```python
from build123d import *

# Parameters (mm, degrees)
EXTRUDE_1_DEPTH     = 5
FILLET_1_R          = 3
SKETCH_11_R         = 2
CUT_EXTRUDE_6_DEPTH = 88.5
SKETCH_12_R         = 2
CUT_EXTRUDE_7_DEPTH = 88.5
SKETCH_13_R         = 1.5
SKETCH_13_R_2       = 9
SKETCH_13_W         = 9.590692188
SKETCH_13_H         = 23
CUT_EXTRUDE_8_DEPTH = 10


with BuildPart() as part:
    # 스케치1 → 보스-돌출1 (new body)
    with BuildSketch(Plane(origin=(0, 0, 0), x_dir=(1, 0, 0), z_dir=(0, 1, 0))):
        Polygon((-60, -30), (-30, -60), (-12.5, -60), (-12.5, -75), (12.5, -75), (12.5, -60), (30, -60), (60, -30), (60, -12.5), (75, -12.5), (75, 12.5), (60, 12.5), (60, 30), (30, 60), (12.5, 60), (12.5, 75), (-12.5, 75), (-12.5, 60), (-30, 60), (-60, 30), (-60, 12.5), (-75, 12.5), (-75, -12.5), (-60, -12.5), align=None)
    extrude(amount=EXTRUDE_1_DEPTH)

    # 필렛1
    fillet_1_edges = [part.edges().sort_by_distance(p)[0] for p in [
        (-12.5, 2.5, -75),
        (12.5, 2.5, -75),
        (75, 2.5, -12.5),
        (75, 2.5, 12.5),
        (12.5, 2.5, 75),
        (-12.5, 2.5, 75),
        (-75, 2.5, 12.5),
        (-75, 2.5, -12.5),
    ]]
    fillet(fillet_1_edges, radius=FILLET_1_R)

    # 스케치11 → 컷-돌출6 (cut, through all)
    with BuildSketch(Plane.XY.offset(12.5)):
        with Locations((-70, 2.5)):
            Circle(SKETCH_11_R)
        with Locations((70, 2.5)):
            Circle(SKETCH_11_R)
    extrude(amount=-CUT_EXTRUDE_6_DEPTH, mode=Mode.SUBTRACT)

    # 스케치12 → 컷-돌출7 (cut, through all)
    with BuildSketch(Plane.ZY.offset(12.5)):
        with Locations((-70, 2.5)):
            Circle(SKETCH_12_R)
        with Locations((70, 2.5)):
            Circle(SKETCH_12_R)
    extrude(amount=-CUT_EXTRUDE_7_DEPTH, mode=Mode.SUBTRACT)

    # 스케치13 → 컷-돌출8 (cut)
    with BuildSketch(Plane(origin=(0, 5, 0), x_dir=(1, 0, 0), z_dir=(0, 1, 0))):
        with Locations((0, 13.85)):
            Circle(SKETCH_13_R)
        with Locations((30, 0)):
            Circle(SKETCH_13_R_2)
        with Locations((0, -13.85)):
            Circle(SKETCH_13_R)
        Rectangle(SKETCH_13_W, SKETCH_13_H)
    extrude(amount=-CUT_EXTRUDE_8_DEPTH, mode=Mode.SUBTRACT)


solid = part.part
```
Verification items for the finished model (mm, model axes). A direction names the side the tool comes from. Give positions to 0.01 mm unless a question says otherwise; leave off trailing zeros. Loops run counter-clockwise (first coordinate to the right, second up) from the corner with the lowest first, then second, coordinate; pieces in that order, holes last. Notation, with made-up numbers: M 55.25,10 L 107.25,10 A12 ccw 107.25,29 Z; hole C -19,83.25 d7. An arc over 180 degrees is marked long. Return JSON: item names as keys, results as strings.
1) Material ranges on L1, parallel to Z at x = 2.5, y = 2.8; L2, parallel to X at y = 3.15, z = 13.85; L3, parallel to X at y = 3.8, z = 0, recorded low to high. Write a range as [from, to].
Findings:
{"L1": "z = [-75, -71.98], [-68.02, -11.5], [11.5, 68.02], [71.98, 75]", "L2": "x = [-60, -1.5], [1.5, 60]", "L3": "x = [-75, -71.52], [-68.48, -4.8], [4.8, 21], [39, 68.48], [71.52, 75]"}
2) Gauge pin test, flat ends, axial feed: P1, Ø2.5, axis at y = 2, z = -66, coming from the -X side; P2, Ø2.5, axis at x = -70, y = 2.5, coming from the -Z side; P3, Ø1.5, axis at x = 6, z = -11.5, coming from the -Y side; P4, Ø1.5, axis at y = 2.5, z = 21, coming from the -X side. Record the tip position at first contact, or that the pin passes through.
Findings:
{"P1": "stops at x = -12.5", "P2": "passes through", "P3": "stops at y = 0", "P4": "stops at x = -60"}
3) Mould release check, pull along X, two halves, no side actions. Record for faces 1 (the flat face through (-60, 2, -21)), 2 (the flat face through (60, 2, -21)), 3 (the flat face through (0, 3, -11.5)): released by +X, released by -X, zero draft, split by the parting line, or undercut.
Findings:
{"face 1": "released by -X", "face 2": "released by +X", "face 3": "undercut"}
4) Tool access check on faces 4 (the flat face through (-12.5, 2, -65)), 5 (the flat face through (12.5, 2, 65)), 6 (the flat face through (-65, 2, 12.5)), 7 (the flat face through (-4.795, 3, 0)). Record the directions out of +Z, -Z, +X, -X, +Y, -Y that give a thin tool (end or side, any length) a straight path to the whole face; none if there is none.
Findings:
{"face 4": "-Z, -X, +Y, -Y", "face 5": "+Z, +X, +Y, -Y", "face 6": "+Z, -X, +Y, -Y", "face 7": "+Y, -Y"}
5) Section check A-A, the plane z = 0. Enter the section's corners in (x, y), and give its area (3 significant figures).
Findings:
{"outline": "M -75,0 L -4.8,0 L -4.8,5 L -75,5 Z; M 4.8,0 L 21,0 L 21,5 L 4.8,5 Z; M 39,0 L 75,0 L 75,5 L 39,5 Z; hole C -70,2.5 d4; hole C 70,2.5 d4", "area": "587 mm2"}
6) Section check B-B, the plane x = 24. Enter the section's corners in (y, z), and give its area (3 significant figures).
Findings:
{"outline": "M 0,-60 L 5,-60 L 5,-6.71 L 0,-6.71 Z; M 0,6.71 L 5,6.71 L 5,60 L 0,60 Z", "area": "533 mm2"}
7) Section check C-C, the plane z = 70. Enter the section's corners in (x, y).
Findings:
{"outline": "M -12.5,0 L 12.5,0 L 12.5,0.5 L -12.5,0.5 Z; M -12.5,4.5 L 12.5,4.5 L 12.5,5 L -12.5,5 Z"}
8) Section check D-D, the plane y = 1.45. Count the separate pieces of the cut face and the enclosed holes in it, and give its area (3 significant figures).
Findings:
{"separate pieces": "5", "enclosed holes": "4", "area": "13,300 mm2"}
